Source: CAD feature listing. Evaluate the final solid. Frame: model axes, mm. Face numbers are marked on the shaded views. A direction names the side the tool comes from. Round coordinates to 2 decimals unless told otherwise and drop trailing zeros. Loops run counter-clockwise (first coordinate to the right, second up) from the corner with the lowest first, then second, coordinate; pieces in that order, holes last.
Item 1: Access query for the marked faces 1, 2, 3, 4 and 5. Directions: +Z, -Z, +X, -X, +Y, -Y. A direction counts if a zero-diameter tool reaches every point of the face in a straight line with its end or side. Return the directions, or none.
Item 2: Ray query, L1, parallel to Z at x = -12, y = 2.05; L2, parallel to Z at x = -10.5, y = 1.1; L3, parallel to X at y = 2.55, z = 9.5. Return the intervals inside material, ascending.
Item 3: Section query D-D on z = -4.25. Return loops of the section in (x, y), then the cut area to 3 significant figures.
Item 4: Section query A-A on z = 11.25. Return loops of the section in (x, y), then the cut area to 3 significant figures.
Item 5: Section query B-B on x = -11.5. Return loops of the section in (y, z).
Item 6: First-contact query: P1, Ø0.9, axis at y = 2, z = 10.5, coming from the +X side; P2, Ø3, axis at x = 0, z = 0, coming from the -Y side; P3, Ø1, axis at y = 0.5, z = 8, coming from the -X side; P4, Ø1, axis at y = 1, z = 7, coming from the +X side. Flat tips, straight axial feed; report the tip coordinate or a pass-through.
Item 7: Section query C-C on x = 5.25. Return loops of the section in (y, z).
Item 8: Pull-direction query (X, two-part tool) for the marked faces 6, 7 and 8; classes: released by +X, released by -X, zero draft, split by the parting line, or undercut.
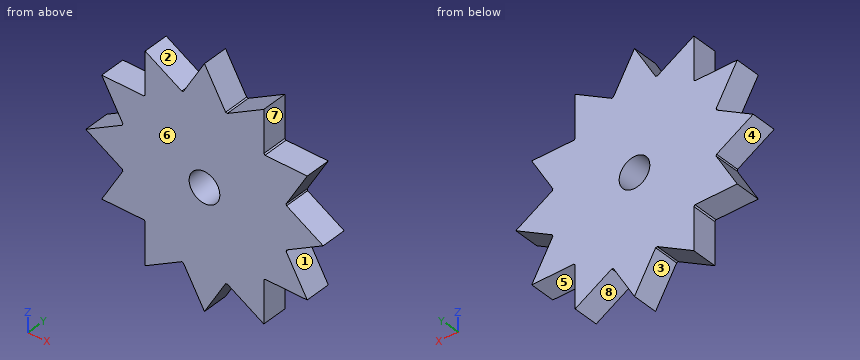
```python
from build123d import *

# Parameters (mm, degrees)
SKETCH1_R           = 10
BOSS_EXTRUDE1_DEPTH = 3
BOSS_EXTRUDE2_DEPTH = 3
CIRPATTERN1_COUNT   = 12
SKETCH3_R           = 1.81
CUT_EXTRUDE1_DEPTH  = 3


with BuildPart() as part:
    # Sketch1 → Boss-Extrude1 (new body)
    with BuildSketch(Plane(origin=(0, 0, 0), x_dir=(1, 0, 0), z_dir=(0, 1, 0))):
        with Locations(Location((0, 0, 0), (0, 0, 270))):
            Circle(SKETCH1_R)
    extrude(amount=BOSS_EXTRUDE1_DEPTH)

    # Sketch2 → Boss-Extrude2 (add)
    with BuildSketch(Plane(origin=(0, 3, 0), x_dir=(1, 0, 0), z_dir=(0, 1, 0))):
        Polygon((0, 14), (-2.491463612, 9.684658438), (2.491463612, 9.684658438), align=None)
    boss_extrude2 = extrude(amount=-BOSS_EXTRUDE2_DEPTH)

    # CirPattern1: Boss-Extrude2 ×12 about axis
    cirpattern1_axis = Axis((0, 0, 0), (0, 1, 0))
    for i in range(1, CIRPATTERN1_COUNT):
        add(boss_extrude2.rotate(cirpattern1_axis, i * 360 / CIRPATTERN1_COUNT))

    # Sketch3 → Cut-Extrude1 (cut)
    with BuildSketch(Plane(origin=(0, 3, 0), x_dir=(1, 0, 0), z_dir=(0, 1, 0))):
        with Locations(Location((0, 0, 0), (0, 0, 270))):
            Circle(SKETCH3_R)
    extrude(amount=-CUT_EXTRUDE1_DEPTH, mode=Mode.SUBTRACT)


solid = part.part
```
Data:
1. face 1: +X, +Y, -Y
1. face 2: +Z, +Y, -Y
1. face 3: -Z, +Y, -Y
1. face 4: -X, +Y, -Y
1. face 5: -Z, +X, +Y, -Y
2. L1: z = -7 to -6.78, -1.15 to 1.15, 6.78 to 7
2. L2: z = -7 to -4.19, -2.02 to 2.02, 4.19 to 7
2. L3: x = -7 to 7
3. outline: (-10.54, 0) - (10.54, 0) - (10.54, 3) - (-10.54, 3) - close
3. area: 63.2 mm2
4. outline: (-7, 0) - (-5.49, 0) - (-5.49, 3) - (-7, 3) - close; (-1.59, 0) - (1.59, 0) - (1.59, 3) - (-1.59, 3) - close; (5.49, 0) - (7, 0) - (7, 3) - (5.49, 3) - close
4. area: 18.6 mm2
5. outline: (0, -7) - (3, -7) - (3, -5.92) - (0, -5.92) - close; (0, -1.44) - (3, -1.44) - (3, 1.44) - (0, 1.44) - close; (0, 5.92) - (3, 5.92) - (3, 7) - (0, 7) - close
6. P1: stops at x = 7
6. P2: passes through
6. P3: stops at x = -7
6. P4: stops at x = 12.12
7. outline: (0, -11.11) - (3, -11.11) - (3, 11.11) - (0, 11.11) - close
8. face 6: zero draft
8. face 7: released by +X
8. face 8: undercut
